The model under review builds one solid part; all positions refer to its coordinate system, in mm. Face numbers are marked on the shaded views. A direction names the side the tool comes from. Coordinates: 2 decimals unless noted, no trailing zeros. Write each loop counter-clockwise with the first axis right and the second up, starting at its lowest first coordinate (ties: lowest second). Pieces come first, ordered by that corner, then holes.
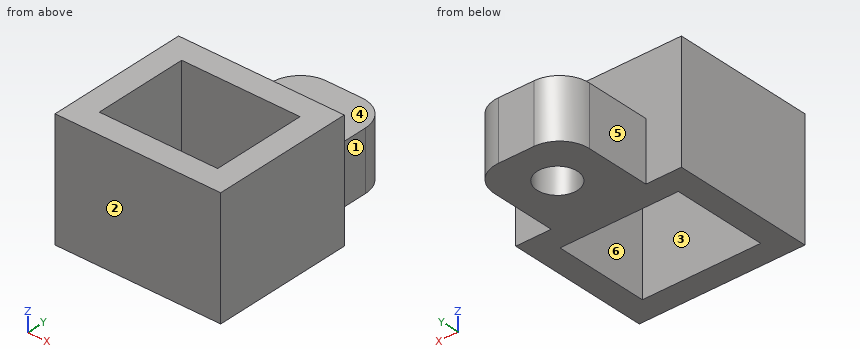
```python
from build123d import *

# Parameters (mm, degrees)
SKETCH2_W           = 14
SKETCH2_H           = 12
BOSS_EXTRUDE1_DEPTH = 10
SKETCH1_W           = 10
SKETCH1_H           = 8
CUT_EXTRUDE2_DEPTH  = 11
SKETCH3_W           = 8
SKETCH3_H           = 8
BOSS_EXTRUDE2_DEPTH = 5
SKETCH4_R           = 1.7
CUT_EXTRUDE3_DEPTH  = 11
FILLET1_R           = 2.5


with BuildPart() as part:
    # Sketch2 → Boss-Extrude1 (new body)
    with BuildSketch(Plane.XY):
        Rectangle(SKETCH2_W, SKETCH2_H)
    extrude(amount=BOSS_EXTRUDE1_DEPTH)

    # Sketch1 → Cut-Extrude2 (cut, through all)
    with BuildSketch(Plane.XY):
        Rectangle(SKETCH1_W, SKETCH1_H)
    extrude(amount=CUT_EXTRUDE2_DEPTH, mode=Mode.SUBTRACT)

    # Sketch3 → Boss-Extrude2 (add)
    with BuildSketch(Plane.XY):
        with Locations((0, 10)):
            Rectangle(SKETCH3_W, SKETCH3_H)
    extrude(amount=BOSS_EXTRUDE2_DEPTH)

    # Sketch4 → Cut-Extrude3 (cut, through all)
    with BuildSketch(Plane.XY):
        with Locations((0, 10)):
            Circle(SKETCH4_R)
    extrude(amount=CUT_EXTRUDE3_DEPTH, mode=Mode.SUBTRACT)

    # Fillet1
    fillet1_edges = [part.edges().sort_by_distance(p)[0] for p in [
        (4, 14, 2.5),
        (-4, 14, 2.5),
    ]]
    fillet(fillet1_edges, radius=FILLET1_R)


solid = part.part
```
Item 1: Take a section at D-D, the plane x = 2.5. Write out the cut boundary in (y, z), plus the area to 3 significant figures.
Solved:
outline: (-6, 0) - (-4, 0) - (-4, 10) - (-6, 10) - close; (4, 0) - (13.79, 0) - (13.79, 5) - (6, 5) - (6, 10) - (4, 10) - close
area: 79.0 mm2
Item 2: Take a section at C-C, the plane z = 4.25. Write out the cut boundary in (x, y), plus the area to 3 significant figures.
Solved:
outline: (-7, -6) - (7, -6) - (7, 6) - (4, 6) - (4, 11.5) arc R2.5 ccw to (1.5, 14) - (-1.5, 14) arc R2.5 ccw to (-4, 11.5) - (-4, 6) - (-7, 6) - close; hole (-5, -4) - (5, -4) - (5, 4) - (-5, 4) - close; hole circle Ø3.4 at (0, 10)
area: 140 mm2
Item 3: Machinability: for the marked faces 4, 5 and 6, which of the approach directions +Z, -Z, +X, -X, +Y, -Y give a long, thin tool a straight path to every point of the face, cutting with its end or side? Answer none if there is none.
Solved:
face 4: +Z, +X, -X, +Y
face 5: +Z, -Z, -X, +Y
face 6: +Z, -Z
Item 4: Take a section at A-A, the plane x = 0. Write out the cut boundary in (y, z).
Solved:
outline: (-6, 0) - (-4, 0) - (-4, 10) - (-6, 10) - close; (4, 0) - (8.3, 0) - (8.3, 5) - (6, 5) - (6, 10) - (4, 10) - close; (11.7, 0) - (14, 0) - (14, 5) - (11.7, 5) - close
Item 5: To check wall thickness, follow line 1 along Y through (x, z) = (0, 1.6); line 2 along X through (y, z) = (10, 1.95); line 3 along Y through (x, z) = (-0.75, 6). State the ranges of each line that lie inside material, in increasing order.
Solved:
line 1: y = -6 to -4, 4 to 8.3, 11.7 to 14
line 2: x = -4 to -1.7, 1.7 to 4
line 3: y = -6 to -4, 4 to 6
Item 6: For pin 1 (1.5 mm diameter, centred on x = 4, z = 5.5, fed in from +Y); pin 2 (2.5 mm diameter, centred on x = 1.5, y = 8.5, fed in from +Z); pin 3 (4 mm diameter, centred on y = 11.5, z = 4, fed in from -X), all flat-tipped, find the tip position at first contact; note any pin that passes through.
Solved:
pin 1: stops at y = 13.08
pin 2: stops at z = 5
pin 3: stops at x = -4
Item 7: Take a section at B-B, the plane y = 10. Write out the cut boundary in (x, z).
Solved:
outline: (-4, 0) - (-1.7, 0) - (-1.7, 5) - (-4, 5) - close; (1.7, 0) - (4, 0) - (4, 5) - (1.7, 5) - close
Item 8: Mouldability with a two-part tool opening along X and no side actions: class the marked faces 1, 2 and 3 as pulls with the +X half, pulls with the -X half, needs draft (parallel to the pull), parting line crosses it, or undercut.
Solved:
face 1: pulls with the +X half
face 2: needs draft
face 3: undercut
